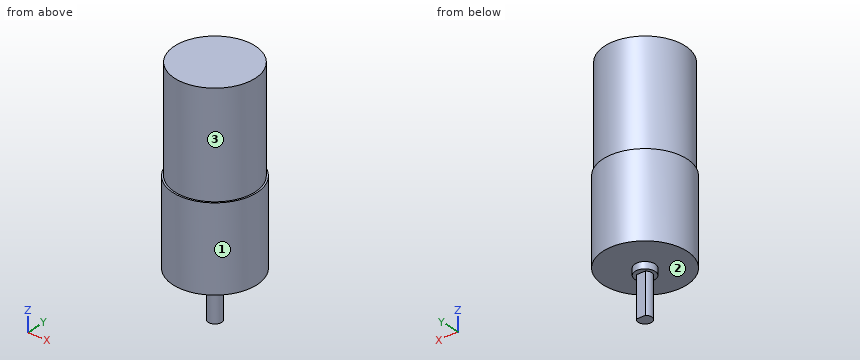
from build123d import *

# Parameters (mm, degrees)
SKETCH1_R           = 12.5
BOSS_EXTRUDE2_DEPTH = 25
SKETCH2_R           = 3
BOSS_EXTRUDE3_DEPTH = 2
SKETCH3_R           = 2
BOSS_EXTRUDE4_DEPTH = 12
CUT_EXTRUDE1_DEPTH  = 12
SKETCH5_R           = 12
BOSS_EXTRUDE5_DEPTH = 30.8


with BuildPart() as part:
    # Sketch1 → Boss-Extrude2 (new body)
    with BuildSketch(Plane.XY):
        Circle(SKETCH1_R)
    extrude(amount=BOSS_EXTRUDE2_DEPTH)

    # Sketch2 → Boss-Extrude3 (add)
    with BuildSketch(Plane(origin=(0, 0, 0), x_dir=(-1, 0, 0), z_dir=(0, 0, -1))):
        Circle(SKETCH2_R)
    extrude(amount=BOSS_EXTRUDE3_DEPTH)

    # Sketch3 → Boss-Extrude4 (add)
    with BuildSketch(Plane(origin=(0, 0, -2), x_dir=(-1, 0, 0), z_dir=(0, 0, -1))):
        Circle(SKETCH3_R)
    extrude(amount=BOSS_EXTRUDE4_DEPTH)

    # Sketch4 → Cut-Extrude1 (cut)
    with BuildSketch(Plane(origin=(0, 0, -14), x_dir=(-1, 0, 0), z_dir=(0, 0, -1))):
        with BuildLine():
            Line((-1.322875656, 1.5), (1.322875656, 1.5))
            ThreePointArc((1.322875656, 1.5), (0, 2), (-1.322875656, 1.5))
        make_face()
    extrude(amount=-CUT_EXTRUDE1_DEPTH, mode=Mode.SUBTRACT)

    # Sketch5 → Boss-Extrude5 (add)
    with BuildSketch(Plane.XY.offset(25)):
        Circle(SKETCH5_R)
    extrude(amount=BOSS_EXTRUDE5_DEPTH)


solid = part.part
Could you check a few things on this model? Use its own coordinates, in mm. Face numbers are marked on the shaded views. A direction names the side the tool comes from. Coordinates: 2 decimals unless noted, no trailing zeros. Write each loop counter-clockwise with the first axis right and the second up, starting at its lowest first coordinate (ties: lowest second). Pieces come first, ordered by that corner, then holes. Notation, with made-up numbers: (70.5, -31) - (97.5, -31) arc R9 ccw to (97.5, -25) - close; hole circle Ø9 at (-14.75, 33.5). An arc over 180 degrees is marked (long way). Write item = value, one per line.
1) Please list where these lines run through material, in increasing order: line 1 (Z direction, x = 4.5, y = 5); line 2 (X direction, y = 0.5, z = 24.5); line 3 (Z direction, x = -11, y = 5.5). Write a range as [from, to].
Result set:
line_1 = [0, 55.8]
line_2 = [-12.49, 12.49]
line_3 = [0, 25]
2) Suppose I cut it at C-C on z = 49. Please give me the cut outline in (x, y), plus the area to 3 significant figures.
Result set:
outline = circle Ø24 at (0, 0)
area = 452 mm2
3) For the marked faces 1, 2 and 3, which set-ups out of +Z, -Z, +X, -X, +Y, -Y let a thin tool reach every point of the face, with its end or its side?
Result set:
face_1 = +Z, -Z
face_2 = -Z
face_3 = +Z
4) Will these pins go through, and if not, where does the flat tip stop? pin 1 Ø2 at (x, z) = (4, 35.5) entering from -Y; pin 2 Ø6 at (x, z) = (-6.5, 33.5) entering from +Y; pin 3 Ø1 at (x, z) = (-6, 31.5) entering from +Y.
Result set:
pin_1 = -11.62
pin_2 = 11.48
pin_3 = 10.67
5) Suppose I cut it at B-B on y = -7.25. Please give me the cut outline in (x, z).
Result set:
outline = (-10.18, 0) - (10.18, 0) - (10.18, 25) - (9.56, 25) - (9.56, 55.8) - (-9.56, 55.8) - (-9.56, 25) - (-10.18, 25) - close
6) Suppose I cut it at D-D on x = 0. Please give me the cut outline in (y, z), plus the area to 3 significant figures.
Result set:
outline = (-12.5, 0) - (-3, 0) - (-3, -2) - (-2, -2) - (-2, -14) - (1.5, -14) - (1.5, -2) - (3, -2) - (3, 0) - (12.5, 0) - (12.5, 25) - (12, 25) - (12, 55.8) - (-12, 55.8) - (-12, 25) - (-12.5, 25) - close
area = 1,420 mm2
7) Suppose I cut it at A-A on x = -4.75. Please give me the cut outline in (y, z), plus the area to 3 significant figures.
Result set:
outline = (-11.56, 0) - (11.56, 0) - (11.56, 25) - (11.02, 25) - (11.02, 55.8) - (-11.02, 55.8) - (-11.02, 25) - (-11.56, 25) - close
area = 1,260 mm2
